Work out the finished part from the listing and answer in its coordinate system (mm). A direction names the side the tool comes from. Round coordinates to 2 decimals unless told otherwise and drop trailing zeros. Return JSON: item names as keys, results as strings.
from build123d import *

# Parameters (mm, degrees)
SKETCH_1_R      = 3.4
EXTRUDE_1_DEPTH = 1000


with BuildPart() as part:
    # Эскиз1 → Бобышка-Вытянуть1 (new body)
    with BuildSketch(Plane.XY):
        with BuildLine():
            Line((5.4, -20), (10.25, -20))
            Line((10.25, -20), (20, -20))
            Line((20, -20), (20, -10.25))
            Line((20, -10.25), (20, -5.4))
            ThreePointArc((20, -5.4), (19.912132034, -5.187867966), (19.7, -5.1))
            Line((19.7, -5.1), (19.3, -5.1))
            ThreePointArc((19.3, -5.1), (19.087867966, -5.012132034), (19, -4.8))
            Line((19, -4.8), (19, -4.4))
            ThreePointArc((19, -4.4), (18.912132034, -4.187867966), (18.7, -4.1))
            Line((18.7, -4.1), (15.8, -4.1))
            ThreePointArc((15.8, -4.1), (15.587867966, -4.187867966), (15.5, -4.4))
            Line((15.5, -4.4), (15.5, -6.3))
            ThreePointArc((15.5, -6.3), (15.587867966, -6.512132034), (15.8, -6.6))
            Line((15.8, -6.6), (17, -6.6))
            ThreePointArc((17, -6.6), (17.707106781, -6.892893219), (18, -7.6))
            Line((18, -7.6), (18, -9.25))
            ThreePointArc((18, -9.25), (17.707106781, -9.957106781), (17, -10.25))
            Line((17, -10.25), (11.664213562, -10.25))
            ThreePointArc((11.664213562, -10.25), (11.28153013, -10.173879533), (10.957106781, -9.957106781))
            Line((10.957106781, -9.957106781), (7.792893219, -6.792893219))
            ThreePointArc((7.792893219, -6.792893219), (7.576120467, -6.46846987), (7.5, -6.085786438))
            Line((7.5, -6.085786438), (7.5, 6.085786438))
            ThreePointArc((7.5, 6.085786438), (7.576120467, 6.46846987), (7.792893219, 6.792893219))
            Line((7.792893219, 6.792893219), (10.957106781, 9.957106781))
            ThreePointArc((10.957106781, 9.957106781), (11.28153013, 10.173879533), (11.664213562, 10.25))
            Line((11.664213562, 10.25), (17, 10.25))
            ThreePointArc((17, 10.25), (17.707106781, 9.957106781), (18, 9.25))
            Line((18, 9.25), (18, 7.6))
            ThreePointArc((18, 7.6), (17.707106781, 6.892893219), (17, 6.6))
            Line((17, 6.6), (15.8, 6.6))
            ThreePointArc((15.8, 6.6), (15.587867966, 6.512132034), (15.5, 6.3))
            Line((15.5, 6.3), (15.5, 4.4))
            ThreePointArc((15.5, 4.4), (15.587867966, 4.187867966), (15.8, 4.1))
            Line((15.8, 4.1), (18.7, 4.1))
            ThreePointArc((18.7, 4.1), (18.912132034, 4.187867966), (19, 4.4))
            Line((19, 4.4), (19, 4.8))
            ThreePointArc((19, 4.8), (19.087867966, 5.012132034), (19.3, 5.1))
            Line((19.3, 5.1), (19.7, 5.1))
            ThreePointArc((19.7, 5.1), (19.912132034, 5.187867966), (20, 5.4))
            Line((20, 5.4), (20, 10.25))
            Line((20, 10.25), (20, 20))
            ThreePointArc((20, 20), (-8.284271247, 8.284271247), (-20, -20))
            Line((-20, -20), (-10.25, -20))
            Line((-10.25, -20), (-5.4, -20))
            ThreePointArc((-5.4, -20), (-5.187867966, -19.912132034), (-5.1, -19.7))
            Line((-5.1, -19.7), (-5.1, -19.3))
            ThreePointArc((-5.1, -19.3), (-5.012132034, -19.087867966), (-4.8, -19))
            Line((-4.8, -19), (-4.4, -19))
            ThreePointArc((-4.4, -19), (-4.187867966, -18.912132034), (-4.1, -18.7))
            Line((-4.1, -18.7), (-4.1, -15.8))
            ThreePointArc((-4.1, -15.8), (-4.187867966, -15.587867966), (-4.4, -15.5))
            Line((-4.4, -15.5), (-6.3, -15.5))
            ThreePointArc((-6.3, -15.5), (-6.512132034, -15.587867966), (-6.6, -15.8))
            Line((-6.6, -15.8), (-6.6, -17))
            ThreePointArc((-6.6, -17), (-6.892893219, -17.707106781), (-7.6, -18))
            Line((-7.6, -18), (-9.25, -18))
            ThreePointArc((-9.25, -18), (-9.957106781, -17.707106781), (-10.25, -17))
            Line((-10.25, -17), (-10.25, -11.664213562))
            ThreePointArc((-10.25, -11.664213562), (-10.173879533, -11.28153013), (-9.957106781, -10.957106781))
            Line((-9.957106781, -10.957106781), (-6.792893219, -7.792893219))
            ThreePointArc((-6.792893219, -7.792893219), (-6.46846987, -7.576120467), (-6.085786438, -7.5))
            Line((-6.085786438, -7.5), (6.085786438, -7.5))
            ThreePointArc((6.085786438, -7.5), (6.46846987, -7.576120467), (6.792893219, -7.792893219))
            Line((6.792893219, -7.792893219), (9.957106781, -10.957106781))
            ThreePointArc((9.957106781, -10.957106781), (10.173879533, -11.28153013), (10.25, -11.664213562))
            Line((10.25, -11.664213562), (10.25, -17))
            ThreePointArc((10.25, -17), (9.957106781, -17.707106781), (9.25, -18))
            Line((9.25, -18), (7.6, -18))
            ThreePointArc((7.6, -18), (6.892893219, -17.707106781), (6.6, -17))
            Line((6.6, -17), (6.6, -15.8))
            ThreePointArc((6.6, -15.8), (6.512132034, -15.587867966), (6.3, -15.5))
            Line((6.3, -15.5), (4.4, -15.5))
            ThreePointArc((4.4, -15.5), (4.187867966, -15.587867966), (4.1, -15.8))
            Line((4.1, -15.8), (4.1, -18.7))
            ThreePointArc((4.1, -18.7), (4.187867966, -18.912132034), (4.4, -19))
            Line((4.4, -19), (4.8, -19))
            ThreePointArc((4.8, -19), (5.012132034, -19.087867966), (5.1, -19.3))
            Line((5.1, -19.3), (5.1, -19.7))
            ThreePointArc((5.1, -19.7), (5.187867966, -19.912132034), (5.4, -20))
        make_face()
        with BuildLine():
            Line((-13.247331922, -18), (-16.878177829, -18))
            ThreePointArc((-16.878177829, -18), (-17.613392451, -17.677834389), (-17.874885338, -16.918918919))
            ThreePointArc((-17.874885338, -16.918918919), (-14.907238495, -4.983852003), (-8.283209505, 5.378338403))
            ThreePointArc((-8.283209505, 5.378338403), (-7.565951428, 5.710121829), (-6.831807736, 5.417594174))
            Line((-6.831807736, 5.417594174), (-5.080320702, 3.66610714))
            ThreePointArc((-5.080320702, 3.66610714), (-4.799630461, 3.114747086), (-4.897054025, 2.503769534))
            ThreePointArc((-4.897054025, 2.503769534), (-5.499751223, -0.052311407), (-4.848542652, -2.596465704))
            ThreePointArc((-4.848542652, -2.596465704), (-4.740862187, -3.21489496), (-5.02298908, -3.775657158))
            Line((-5.02298908, -3.775657158), (-12.247331922, -11))
            Line((-12.247331922, -11), (-12.247331922, -17))
            ThreePointArc((-12.247331922, -17), (-12.540225141, -17.707106781), (-13.247331922, -18))
        make_face(mode=Mode.SUBTRACT)
        with BuildLine():
            ThreePointArc((12.2, -13.2), (12.492893219, -12.492893219), (13.2, -12.2))
            Line((13.2, -12.2), (17, -12.2))
            ThreePointArc((17, -12.2), (17.707106781, -12.492893219), (18, -13.2))
            Line((18, -13.2), (18, -17))
            ThreePointArc((18, -17), (17.707106781, -17.707106781), (17, -18))
            Line((17, -18), (13.2, -18))
            ThreePointArc((13.2, -18), (12.492893219, -17.707106781), (12.2, -17))
            Line((12.2, -17), (12.2, -13.2))
        make_face(mode=Mode.SUBTRACT)
        Circle(SKETCH_1_R, mode=Mode.SUBTRACT)
        with BuildLine():
            Line((-3.66610714, 5.080320702), (-5.417594174, 6.831807736))
            ThreePointArc((-5.417594174, 6.831807736), (-5.710121829, 7.565951428), (-5.378338403, 8.283209505))
            ThreePointArc((-5.378338403, 8.283209505), (4.983852003, 14.907238495), (16.918918919, 17.874885338))
            ThreePointArc((16.918918919, 17.874885338), (17.677834389, 17.613392451), (18, 16.878177829))
            Line((18, 16.878177829), (18, 13.247331922))
            ThreePointArc((18, 13.247331922), (17.707106781, 12.540225141), (17, 12.247331922))
            Line((17, 12.247331922), (11, 12.247331922))
            Line((11, 12.247331922), (3.775657158, 5.02298908))
            ThreePointArc((3.775657158, 5.02298908), (3.21489496, 4.740862187), (2.596465704, 4.848542652))
            ThreePointArc((2.596465704, 4.848542652), (0.052311407, 5.499751223), (-2.503769534, 4.897054025))
            ThreePointArc((-2.503769534, 4.897054025), (-3.114747086, 4.799630461), (-3.66610714, 5.080320702))
        make_face(mode=Mode.SUBTRACT)
    extrude(amount=EXTRUDE_1_DEPTH)


solid = part.part
Item 1: Consider line 1 along Y through (x, z) = (16, 898); line 2 along Y through (x, z) = (12, 915); line 3 along Y through (x, z) = (0, 480). Determine where each line is inside the solid, lowest interval first. Write a range as [from, to].
Output:
{"line 1": "y = [-20, -18], [-12.2, -10.25], [-6.6, -4.1], [4.1, 6.6], [10.25, 12.25], [17.79, 19.8]", "line 2": "y = [-20, -10.25], [10.25, 12.25], [17.15, 19.19]", "line 3": "y = [-7.5, -3.4], [3.4, 5.5], [12.31, 14.64]"}
Item 2: Find section A-A (z = 502). State how many separate pieces and enclosed holes the cut face has, plus the area to 3 significant figures.
Output:
{"separate pieces": "1", "enclosed holes": "4", "area": "482 mm^2"}
Item 3: Which of the six approach directions +Z, -Z, +X, -X, +Y, -Y give full straight-line access (tool end or side, diameter ignored) to faces 4 (the cylindrical face through (4.83, 14.84, 493)), 5 (the flat face through (3, -4, 1000))?
Output:
{"face 4": "+Z, -Z", "face 5": "+Z, +X, -X, +Y, -Y"}
Item 4: The mould has two halves that part along Y. Classify faces 1 (the cylindrical face through (-14.975, -5.143, 493)), 2 (the flat face through (3, -4, 0)), 3 (the cylindrical face through (-7.972, 8.594, 493)): pulls with the +Y half, pulls with the -Y half, needs draft (parallel to the pull), parting line crosses it, or undercut.
Output:
{"face 1": "undercut", "face 2": "needs draft", "face 3": "pulls with the +Y half"}
Item 5: Each of these flat-tipped pins is pushed along its axis until it touches: pin 1 (1.8 mm diameter, centred on y = 16, z = 569, fed in from -X); pin 2 (1.5 mm diameter, centred on y = 10, z = 325.5, fed in from -X); pin 3 (12 mm diameter, centred on x = 10, z = 846, fed in from +Y). Where does it stop, or does it pass through?
Output:
{"pin 1": "stops at x = 0.82", "pin 2": "stops at x = -7.28", "pin 3": "stops at y = 19.8"}
